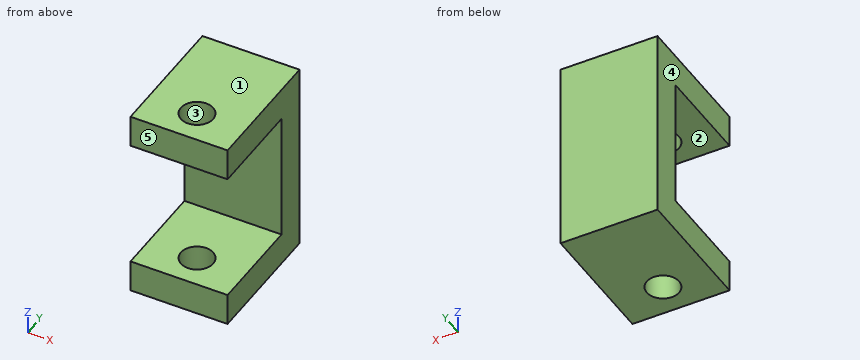
Autodesk Inventor part; units mm, degrees
ref_plane "YZ Plane" through (0, 0, 0) normal (1, 0, 0) x (0, 1, 0)
ref_plane "XZ Plane" through (0, 0, 0) normal (0, 1, 0) x (-1, 0, 0)
ref_plane "XY Plane" through (0, 0, 0) normal (0, 0, 1) x (1, 0, 0)
sketch "Эскиз1" plane through (0, 0, 0) normal (0, 0, 1) x (1, 0, 0)
  line L0 (0, 0) -> (15, 0)
  line L1 (15, 0) -> (15, 20)
  line L2 (15, 20) -> (0, 20)
  line L3 (0, 20) -> (0, 0)
  dimension "d0" = 15
  dimension "d1" = 20
extrude "Выдавливание1" add sketch "Эскиз1" along normal blind 5
sketch "Эскиз2" plane through (0, 0, 5) normal (0, 0, 1) x (1, 0, 0)
  line L0 (0, 20) -> (0, 0)
  line L1 (15, 0) -> (15, 20)
  line L2 (0, 20) -> (15, 20)
  line L3 (15, 20) -> (15, 15)
  line L4 (15, 15) -> (0, 15)
  line L5 (0, 15) -> (0, 20)
  point P0 (15, 20)
  point P1 (0, 15)
  dimension "d4" = 5
extrude "Выдавливание2" add sketch "Эскиз2" along normal blind 10
mirror "Зеркальное отражение1" about plane through (7.5, 17.5, 15) normal (0, 0, 1) of "Выдавливание2", "Выдавливание1"
sketch "Эскиз3" plane through (0, 0, 5) normal (0, 0, 1) x (1, 0, 0)
  line L0 (0, 0) -> (15, 0)
  line L1 (7.5, 0) -> (7.5, 5)
  dimension "d7" = 5
hole "Отверстие1" at (7.5, 5, 5) direction (0, 0, -1) diameter 5 end through all both
properties part number "Поворотный рычаг"
Model file for the job. Use its own axes, mm. Face numbers are marked on the shaded views. A direction names the side the tool comes from. Give positions to 0.01 mm unless a question says otherwise; leave off trailing zeros. Loops run counter-clockwise (first coordinate to the right, second up) from the corner with the lowest first, then second, coordinate; pieces in that order, holes last.
1) Saw through at B-B (y = 10.5). Write the cut outline in (x, z), plus the area to 3 significant figures.
2) Tool access for the marked faces 1 and 2: list every direction of +Z, -Z, +X, -X, +Y, -Y with a clear straight run to the whole face (end or side of a thin tool).
3) Pull direction Y, two halves, no side cores. Call the marked faces 3, 4 and 5: +Y half, -Y half, draft (parallel to the pull), parting line (faces both ways), or undercut.
4) Saw through at D-D (x = 2.75). Write the cut outline in (y, z).
5) Saw through at C-C (y = 5). Write the cut outline in (x, z).
6) Saw through at A-A (x = 9). Write the cut outline in (y, z), plus the area to 3 significant figures.
7) Wall check: line 1 (Y direction, x = 7.5, z = 28.6); line 2 (Z direction, x = 1, y = 11); line 3 (X direction, y = 5, z = 2.5). Give the ranges that are in metal, low to high.
Answer block:
1. outline: (0, 0) - (15, 0) - (15, 5) - (0, 5) - close; (0, 25) - (15, 25) - (15, 30) - (0, 30) - close
1. area: 150 mm2
2. face 1: +Z, +X, -X, +Y, -Y
2. face 2: +X, -X, -Y
3. face 3: undercut
3. face 4: draft
3. face 5: -Y half
4. outline: (0, 0) - (20, 0) - (20, 30) - (0, 30) - (0, 25) - (15, 25) - (15, 5) - (0, 5) - close
5. outline: (0, 0) - (5, 0) - (5, 5) - (0, 5) - close; (0, 25) - (5, 25) - (5, 30) - (0, 30) - close; (10, 0) - (15, 0) - (15, 5) - (10, 5) - close; (10, 25) - (15, 25) - (15, 30) - (10, 30) - close
6. outline: (0, 0) - (3, 0) - (3, 5) - (0, 5) - close; (0, 25) - (3, 25) - (3, 30) - (0, 30) - close; (7, 0) - (20, 0) - (20, 30) - (7, 30) - (7, 25) - (15, 25) - (15, 5) - (7, 5) - close
6. area: 260 mm2
7. line 1: y = 0 to 2.5, 7.5 to 20
7. line 2: z = 0 to 5, 25 to 30
7. line 3: x = 0 to 5, 10 to 15
